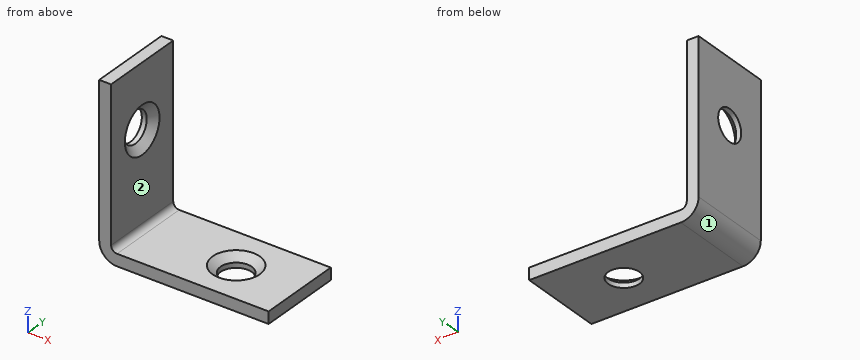
from build123d import *

# Parameters (mm, degrees)
EXTRUDE_THIN1_START = -6.35
EXTRUDE_THIN1_DEPTH = 12.7
SKETCH4_R           = 2.3495
EXTRUDE3_DEPTH      = 33.79453796
CIRPATTERN1_COUNT   = 2


# Read off the part's stored shape, not the designer's step: Extrude-Thin1
with BuildPart() as part:
    # Extrude-Thin1 outline → Extrude-Thin1 (new body)
    with BuildSketch(Plane(origin=(0, 0, 0), x_dir=(1, 0, 0), z_dir=(0, 1, 0)).offset(EXTRUDE_THIN1_START)):
        with BuildLine():
            Line((2.667, -1.778), (25.4, -1.778))
            Line((25.4, -1.778), (25.4, 0))
            Line((25.4, 0), (2.667, 0))
            ThreePointArc((2.667, 0), (0.781146215, -0.781146215), (0, -2.667))
            Line((0, -2.667), (0, -25.4))
            Line((0, -25.4), (1.778, -25.4))
            Line((1.778, -25.4), (1.778, -2.667))
            ThreePointArc((1.778, -2.667), (2.038382072, -2.038382072), (2.667, -1.778))
        make_face()
    extrude(amount=EXTRUDE_THIN1_DEPTH)

    # Sketch4 → Extrude3 (cut, through all)
    with BuildSketch(Plane(origin=(3.556, 0, 1.778), x_dir=(1, 0, 0), z_dir=(0, 0, 1))):
        with Locations((12.319, 0)):
            Circle(SKETCH4_R)
        with Locations((-13.081, 0)):
            Circle(SKETCH4_R)
        with Locations((-38.481, 0)):
            Circle(SKETCH4_R)
        with Locations((-63.881, 0)):
            Circle(SKETCH4_R)
    extrude3 = extrude(amount=-EXTRUDE3_DEPTH, mode=Mode.SUBTRACT)

    # Cut-Extrude1 cone 1 section (through the dimple's axis) → Cut-Extrude1 (revolve, cut)
    with BuildSketch(Plane(origin=(15.875, 0, 1.778), x_dir=(0, -1, 0), z_dir=(1, 0, 0))):
        Polygon((0, 0), (3.5433, 0), (0, 3.080143698), align=None)
    cut_extrude1 = revolve(axis=Axis((15.875, 0, 1.778), (0, 0, -1)), mode=Mode.SUBTRACT)

    # CirPattern1: Extrude3, Cut-Extrude1 ×2 about axis
    cirpattern1_axis = Axis((0, 0, 0), (0.7071067811865464, 0, 0.7071067811865487))
    add([extrude3.rotate(cirpattern1_axis, i * 360 / CIRPATTERN1_COUNT) for i in range(1, CIRPATTERN1_COUNT)], mode=Mode.SUBTRACT)
    add([cut_extrude1.rotate(cirpattern1_axis, i * 360 / CIRPATTERN1_COUNT) for i in range(1, CIRPATTERN1_COUNT)], mode=Mode.SUBTRACT)


solid = part.part
Verification items for the finished model (mm, model axes). Face numbers are marked on the shaded views. A direction names the side the tool comes from. Coordinates: 2 decimals unless noted, no trailing zeros. Loops run counter-clockwise (first coordinate to the right, second up) from the corner with the lowest first, then second, coordinate; pieces in that order, holes last. Notation, with made-up numbers: (25, -3.5) -> (51, -3.5) arc R26 ccw to (51, 29.5) -> close; hole circle Ø5 at (88.25, 3.5). An arc over 180 degrees is marked (long way). Answer as a JSON object with one key per item and string values. Group by question number.
Item 1: Depth check by flat-ended pin: pin 1 (3 mm diameter, centred on x = 23, z = 4, fed in from +Y) (3 decimals); pin 2 (3 mm diameter, centred on x = 18, y = 3, fed in from -Z); pin 3 (4 mm diameter, centred on x = 12.5, y = 2.5, fed in from +Z); pin 4 (6 mm diameter, centred on y = 0, z = 15.875, fed in from +X). Enter the tip coordinate at first touch or a pass-through.
Item 2: Sectioned sample at C-C on x = 4. Record the boundary of the cut face in (y, z), plus the area to 3 significant figures.
Item 3: Sectioned sample at A-A on y = 0. Record the boundary of the cut face in (x, z).
Item 4: Tool access check on the marked faces 1 and 2. Record the directions out of +Z, -Z, +X, -X, +Y, -Y that give a thin tool (end or side, any length) a straight path to the whole face; none if there is none.
Item 5: Sectioned sample at B-B on y = 5. Record the boundary of the cut face in (x, z).
Item 6: Scan lines: probe 1 along X at (y, z) = (2, 5); probe 2 along X at (y, z) = (0, 0.5). Record each from-to range of solid material in increasing order.
Item 7: Sectioned sample at D-D on z = 10.5. Record the boundary of the cut face in (x, y), plus the area to 3 significant figures.
Evaluation:
{
 "1": {"pin 1": "passes through", "pin 2": "stops at z = 0", "pin 3": "stops at z = 1.78", "pin 4": "stops at x = 1.31"},
 "2": {"outline": "(-6.35, 0) -> (6.35, 0) -> (6.35, 1.78) -> (-6.35, 1.78) -> close", "area": "22.6 mm²"},
 "3": {"outline": "(0, 2.67) arc R2.67 ccw to (2.67, 0) -> (13.53, 0) -> (13.53, 0.74) -> (12.33, 1.78) -> (2.67, 1.78) arc R0.89 cw to (1.78, 2.67) -> (1.78, 12.33) -> (0.74, 13.53) -> (0, 13.53) -> close; (0, 18.22) -> (0.74, 18.22) -> (1.78, 19.42) -> (1.78, 25.4) -> (0, 25.4) -> close; (18.22, 0) -> (25.4, 0) -> (25.4, 1.78) -> (19.42, 1.78) -> (18.22, 0.74) -> close"},
 "4": {"face 1": "-Z, -X, +Y, -Y", "face 2": "+Z, +X, +Y, -Y"},
 "5": {"outline": "(0, 2.67) arc R2.67 ccw to (2.67, 0) -> (25.4, 0) -> (25.4, 1.78) -> (2.67, 1.78) arc R0.89 cw to (1.78, 2.67) -> (1.78, 25.4) -> (0, 25.4) -> close"},
 "6": {"probe 1": "x = 0 to 1.78", "probe 2": "x = 1.11 to 13.53, 18.22 to 25.4"},
 "7": {"outline": "(0, -6.35) -> (1.78, -6.35) -> (1.78, 6.35) -> (0, 6.35) -> close", "area": "22.6 mm²"}
}
